Check sheet for the modelled part. Datum: model origin and axes. Units: mm. Round coordinates to 2 decimals unless told otherwise and drop trailing zeros. Write each loop counter-clockwise with the first axis right and the second up, starting at its lowest first coordinate (ties: lowest second). Pieces come first, ordered by that corner, then holes. Notation, with made-up numbers: (-22, 27.5) -> (31, 27.5) arc R4 ccw to (31, 33.5) -> close; hole circle Ø2 at (-35, -6.75). An arc over 180 degrees is marked (long way). Write item = value, one per line.
from build123d import *

# Parameters (mm, degrees)
EXTRUDE_THIN1_DEPTH = 261.9375
FILLET1_R           = 0.889


with BuildPart() as part:
    # Sketch1 → Extrude-Thin1 (new body)
    with BuildSketch(Plane.XY):
        with BuildLine():
            Line((-0.333026442, 4.7625), (0, 0))
            Line((0, 0), (-3.96875, 0))
            ThreePointArc((-3.96875, 0), (-4.818557487, 5.609954997), (-8.7077172, 9.741323362))
            ThreePointArc((-8.7077172, 9.741323362), (-11.842464504, 13.007739441), (-12.649448407, 17.4625))
            Line((-12.649448407, 17.4625), (-15.08125, 17.4625))
            Line((-15.08125, 17.4625), (-15.08125, 26.19375))
            Line((-15.08125, 26.19375), (-9.525, 25.805219151))
            Line((-9.525, 25.805219151), (-7.540625, 23.677237492))
            Line((-7.540625, 23.677237492), (-5.55625, 25.527697116))
            Line((-5.55625, 25.527697116), (-4.949953458, 24.877523675))
            Line((-4.949953458, 24.877523675), (-7.584501899, 22.420767509))
            Line((-7.584501899, 22.420767509), (-9.936346881, 24.94281248))
            Line((-9.936346881, 24.94281248), (-14.19225, 25.240414217))
            Line((-14.19225, 25.240414217), (-14.19225, 18.3515))
            Line((-14.19225, 18.3515), (-11.579833127, 18.3515))
            ThreePointArc((-11.579833127, 18.3515), (-11.263384071, 13.868774929), (-8.271283672, 10.515821118))
            ThreePointArc((-8.271283672, 10.515821118), (-4.255672213, 6.4560014), (-2.984543996, 0.889))
            Line((-2.984543996, 0.889), (-0.953335783, 0.889))
            Line((-0.953335783, 0.889), (-1.219860883, 4.700486495))
            Line((-1.219860883, 4.700486495), (-0.333026442, 4.7625))
        make_face()
    extrude(amount=-EXTRUDE_THIN1_DEPTH)

    # Fillet1
    fillet1_edges = [part.edges().sort_by_distance(p)[0] for p in [
        (-7.584501899, 22.420767509, -130.96875),
        (-11.579833127, 18.3515, -130.96875),
        (0, 0, -130.96875),
        (-3.96875, 0, -130.96875),
        (-15.08125, 17.4625, -130.96875),
        (-15.08125, 26.19375, -130.96875),
        (-9.525, 25.805219151, -130.96875),
    ]]
    fillet(fillet1_edges, radius=FILLET1_R)


solid = part.part
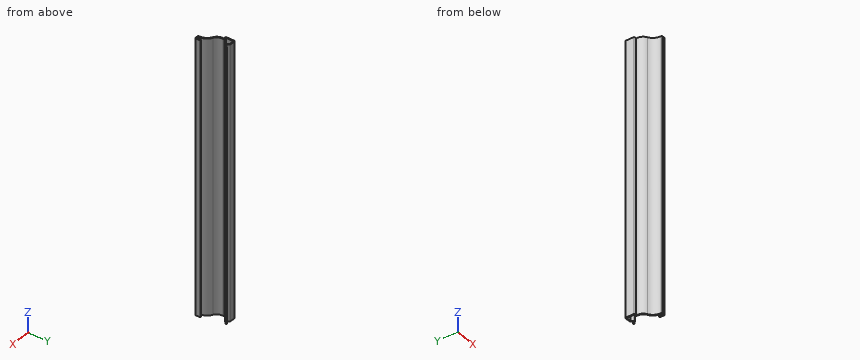
(1) Material ranges on L1, parallel to X at y = 24, z = -97.5; L2, parallel to X at y = 22, z = -180.5; L3, parallel to X at y = 3.25, z = -199, recorded low to high. Write a range as [from, to].
Worked answers:
L1 = [-15.08, -14.19], [-9.06, -7.84], [-7.19, -5.89]
L2 = [-15.08, -14.19]
L3 = [-4.03, -3.13], [-1.12, -0.23]
(2) Sectioned sample at B-B on y = 7.5. Enter the section's corners in (x, z), then the cut area to 3 significant figures.
Worked answers:
outline = (-6.03, -261.94) -> (-4.91, -261.94) -> (-4.91, 0) -> (-6.03, 0) -> close
area = 293 mm²
(3) Go/stop test with flat-tipped pins: P1, Ø6, axis at x = -12.5, z = -106.5, coming from the +Y side; P2, Ø5.5, axis at y = 21.5, z = -123, coming from the +X side; P3, Ø1, axis at x = -7, y = 21, coming from the -Z side; P4, Ø4, axis at x = -11, z = -85, coming from the -Y side. Record where each tip stops, or that it passes through.
Worked answers:
P1 = 26.13
P2 = -5.62
P3 = through
P4 = 9.91
